from build123d import *

# Parameters (mm, degrees)
F0_W     = 52.324
F0_H     = 152.4
F1_DEPTH = 76.2
F3_DEPTH = 142.494
F4_R     = 23.495
F5_DEPTH = 4.826
F6_R     = 9.525
F7_DEPTH = 55.372
F8_R     = 4.7625
F9_DEPTH = 12.7


with BuildPart() as f1:
    # F0 (on Top) → F1 (new body)
    with BuildSketch(Plane.XY):
        with Locations((26.162, 76.2)):
            Rectangle(F0_W, F0_H)
    extrude(amount=F1_DEPTH)

    # F2 (on face) → F3 (join)
    with BuildSketch(Plane.YZ.offset(52.324)):
        with BuildLine():
            Line((152.4, 31.89907), (152.4, 44.30093))
            ThreePointArc((152.4, 44.30093), (139.459111, 67.15052), (114.808, 76.2))
            ThreePointArc((114.808, 76.2), (76.708, 38.1), (114.808, 0))
            ThreePointArc((114.808, 0), (139.459111, 9.04948), (152.4, 31.89907))
        make_face()
    extrude(amount=F3_DEPTH)

    # F4 (on face) → F5 (join)
    with BuildSketch(Plane(origin=(0, 0, 0), x_dir=(0, -1, 0), z_dir=(-1, 0, 0))):
        with Locations((-40.695388, 37.154574)):
            Circle(F4_R)
    extrude(amount=F5_DEPTH)

    # F6 (on face) → F7 (join)
    with BuildSketch(Plane(origin=(-4.826, 0, 0), x_dir=(0, -1, 0), z_dir=(-1, 0, 0))):
        with Locations((-40.695388, 37.154574)):
            Circle(F6_R)
    extrude(amount=F7_DEPTH)

    # F8 (on face) → F9 (join)
    with BuildSketch(Plane.YZ.offset(194.818)):
        with Locations((114.808, 38.1)):
            Circle(F8_R)
    extrude(amount=F9_DEPTH)


solid = f1.part
Check sheet for the modelled part. Datum: model origin and axes. Units: mm. A direction names the side the tool comes from. Give positions to 0.01 mm unless a question says otherwise; leave off trailing zeros. Order: outer loops, then holes, each group sorted by start corner. A loop starts at its lowest first (then second) coordinate and runs counter-clockwise, first axis right, second up. Notation, with made-up numbers: M 79,39.5 L 89,39.5 A11 ccw 89,55.5 Z; hole C 15.5,62 d2. An arc over 180 degrees is marked long. Answer as CSV lines item,"result". Start each with the question number.
Item 1: Cross-section at C-C on x = -26.5. Enter the section's corners in (y, z) (3 decimals).
Item 2: Gauge pin test, flat ends, axial feed: P1, Ø8, axis at y = 122.5, z = 37.5, coming from the -X side; P2, Ø9.5, axis at y = 133, z = 13.5, coming from the +X side; P3, Ø1, axis at y = 30.5, z = 68.5, coming from the +X side. Record the tip position at first contact, or that the pin passes through.
Item 3: Tool access check on faces 1 (the face through (201.08, 119.21, 36.28)), 2 (the face through (-4.826, 41, 27)), 3 (the face through (52.324, 143, 8)), 4 (the face through (52.324, 143, 68)), 5 (the face through (26, 0, 38)). Record the directions out of +Z, -Z, +X, -X, +Y, -Y that give a thin tool (end or side, any length) a straight path to the whole face; none if there is none.
Item 4: Thickness scan on line 1 (X direction, y = 19, z = 45); line 2 (X direction, y = 10, z = 6); line 3 (Y direction, x = 90, z = 37). Record the ranges inside material, lowest first. Write a range as [from, to].
Item 5: Cross-section at D-D on z = 51. Enter the section's corners in (x, y).
Item 6: Cross-section at B-B on y = 58. Enter the section's corners in (x, z).
Item 7: Cross-section at A-A on z = 24. Enter the section's corners in (x, y).
Established:
1,outline,"C 40.695,37.155 d19.05"
2,P1,"stops at x = 0"
2,P2,"stops at x = 194.82"
2,P3,"stops at x = 52.32"
3,face 1,"+X"
3,face 2,"-X"
3,face 3,"-Z, +X, +Y"
3,face 4,"+Z, +X, +Y"
3,face 5,"+Z, -Z, +X, -X, -Y"
4,line 1,"x = [-4.83, 52.32]"
4,line 2,"x = [0, 52.32]"
4,line 3,"y = [76.72, 152.4]"
5,outline,"M -4.83,21.71 L 0,21.71 L 0,0 L 52.32,0 L 52.32,78.96 L 194.82,78.96 L 194.82,150.66 L 52.32,150.66 L 52.32,152.4 L 0,152.4 L 0,59.68 L -4.83,59.68 Z"
6,outline,"M -4.83,21.26 L 0,21.26 L 0,0 L 52.32,0 L 52.32,76.2 L 0,76.2 L 0,53.05 L -4.83,53.05 Z"
7,outline,"M -4.83,21.23 L 0,21.23 L 0,0 L 52.32,0 L 52.32,79.41 L 194.82,79.41 L 194.82,150.2 L 52.32,150.2 L 52.32,152.4 L 0,152.4 L 0,60.16 L -4.83,60.16 Z"
